The listing builds one solid part. Answer for the finished solid, in the listing's coordinates (mm). Face numbers are marked on the shaded views. A direction names the side the tool comes from. Coordinates: 2 decimals unless noted, no trailing zeros. Write each loop counter-clockwise with the first axis right and the second up, starting at its lowest first coordinate (ties: lowest second). Pieces come first, ordered by that corner, then holes.
(1) Straight lines are drawn through the part: line 1 (X direction, y = -2.05, z = 10.5); line 2 (X direction, y = -4.45, z = 26.5); line 3 (Z direction, x = 48, y = -2.05). For each, find the intervals that lie inside material, in ascending order.
(2) For a pull along X with two mould halves and no side action, classify the marked faces 1, 2, 3 and 4 as +X half, -X half, draft (parallel to the pull), parting line (faces both ways), or undercut.
(3) The part is cut by section C-C on z = 10.25. Determine the outline of the cut face in (x, y), plus the area to 3 significant figures.
(4) Given P1, Ø4, axis at x = 16.5, z = 9.5, coming from the +Y side; P2, Ø10, axis at x = 13.09, z = 10.66, coming from the +Y side, each flat-ended and moving along its own axis, determine where each tip first touches the part or whether it passes through.
(5) The part is cut by section B-B on x = 1.5. Determine the outline of the cut face in (y, z), plus the area to 3 significant figures.
(6) The part is cut by section D-D on x = 32.5. Determine the outline of the cut face in (y, z), plus the area to 3 significant figures.
(7) The part is cut by section A-A on z = 22.25. Determine the outline of the cut face in (x, y).
(8) Which of the six approach directions +Z, -Z, +X, -X, +Y, -Y give full straight-line access (tool end or side, diameter ignored) to the marked faces 5, 6 and 7?
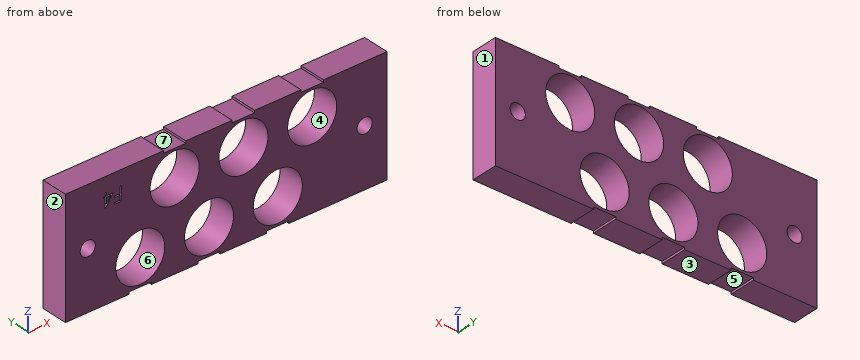
from build123d import *

# Parameters (mm, degrees)
SKETCH1_R               = 5.5
BOSS_EXTRUDE1_DEPTH     = 6
BOSS_EXTRUDE1_2_DEPTH   = 6
BOSS_EXTRUDE1_3_DEPTH   = 6
BOSS_EXTRUDE1_4_DEPTH   = 6
BOSS_EXTRUDE1_5_DEPTH   = 6
BOSS_EXTRUDE1_6_DEPTH   = 6
BOSS_EXTRUDE2_START     = -6
BOSS_EXTRUDE2_OUTLINE_R = 1.7
BOSS_EXTRUDE2_DEPTH     = 6
CUT_EXTRUDE1_DEPTH      = 1


# Read off the part's stored shape, not the designer's step: Boss-Extrude2
with BuildPart() as part:
    # Sketch1 → Boss-Extrude1 (new body)
    with BuildSketch(Plane(origin=(0, 0, 0), x_dir=(1, 0, 0), z_dir=(0, 1, 0))):
        Polygon((3.686387934, -16.664883738), (3.686388262, -4.664883738), (-8.313611738, -4.66488341), (-8.313612066, -16.66488341), align=None)
        with Locations(Location((-2.313611902, -10.664883574, 0), (0, 0, 270))):
            Circle(SKETCH1_R, mode=Mode.SUBTRACT)
    extrude(amount=-BOSS_EXTRUDE1_DEPTH)



with BuildPart() as body_2:
    # Sketch1 → Boss-Extrude1 2 (new body)
    with BuildSketch(Plane(origin=(0, 0, 0), x_dir=(1, 0, 0), z_dir=(0, 1, 0))):
        Polygon((19.086387939, -16.664884095), (19.086388267, -4.664884095), (7.086388267, -4.664883767), (7.086387939, -16.664883767), align=None)
        with Locations(Location((13.086388103, -10.664883931, 0), (0, 0, 270))):
            Circle(SKETCH1_R, mode=Mode.SUBTRACT)
    extrude(amount=-BOSS_EXTRUDE1_2_DEPTH)


with BuildPart() as body_3:
    # Sketch1 → Boss-Extrude1 3 (new body)
    with BuildSketch(Plane(origin=(0, 0, 0), x_dir=(1, 0, 0), z_dir=(0, 1, 0))):
        Polygon((34.486387949, -16.66488445), (34.486388277, -4.66488445), (22.486388277, -4.664884122), (22.486387949, -16.664884122), align=None)
        with Locations(Location((28.486388113, -10.664884286, 0), (0, 0, 270))):
            Circle(SKETCH1_R, mode=Mode.SUBTRACT)
    extrude(amount=-BOSS_EXTRUDE1_3_DEPTH)


with BuildPart() as body_4:
    # Sketch1 → Boss-Extrude1 4 (new body)
    with BuildSketch(Plane(origin=(0, 0, 0), x_dir=(1, 0, 0), z_dir=(0, 1, 0))):
        Polygon((14.786387887, -17.664883977), (14.786387559, -29.664883977), (26.786387559, -29.664884305), (26.786387887, -17.664884305), align=None)
        with Locations(Location((20.786387723, -23.664884141, 0), (0, 0, 270))):
            Circle(SKETCH1_R, mode=Mode.SUBTRACT)
    extrude(amount=-BOSS_EXTRUDE1_4_DEPTH)


with BuildPart() as body_5:
    # Sketch1 → Boss-Extrude1 5 (new body)
    with BuildSketch(Plane(origin=(0, 0, 0), x_dir=(1, 0, 0), z_dir=(0, 1, 0))):
        Polygon((30.186386338, -17.664884333), (30.18638601, -29.664884333), (42.18638601, -29.664884661), (42.186386338, -17.664884661), align=None)
        with Locations(Location((36.186386174, -23.664884497, 0), (0, 0, 270))):
            Circle(SKETCH1_R, mode=Mode.SUBTRACT)
    extrude(amount=-BOSS_EXTRUDE1_5_DEPTH)


with BuildPart() as body_6:
    # Sketch1 → Boss-Extrude1 6 (new body)
    with BuildSketch(Plane(origin=(0, 0, 0), x_dir=(1, 0, 0), z_dir=(0, 1, 0))):
        Polygon((-0.613612103, -17.664883618), (-0.613612431, -29.664883618), (11.386387569, -29.664883947), (11.386387897, -17.664883947), align=None)
        with Locations(Location((5.386387733, -23.664883782, 0), (0, 0, 270))):
            Circle(SKETCH1_R, mode=Mode.SUBTRACT)
    extrude(amount=-BOSS_EXTRUDE1_6_DEPTH)


with BuildPart() as part_1:
    add(part.part)

    add(body_2.part)  # Boss-Extrude2 merges body 2

    add(body_3.part)  # Boss-Extrude2 merges body 3

    add(body_4.part)  # Boss-Extrude2 merges body 4

    add(body_5.part)  # Boss-Extrude2 merges body 5

    add(body_6.part)  # Boss-Extrude2 merges body 6
    # Boss-Extrude2 outline → Boss-Extrude2 (add)
    with BuildSketch(Plane(origin=(0, 0, 0), x_dir=(1, 0, 0), z_dir=(0, 1, 0)).offset(BOSS_EXTRUDE2_START)):
        Polygon((10.586388281, -4.164883862), (0.186388276, -4.164883578), (0.186388262, -4.664883642), (3.686388262, -4.664883738), (3.686387934, -16.664883738), (-8.313612066, -16.66488341), (-8.313611738, -4.66488341), (-4.813611738, -4.664883506), (-4.813611724, -4.164883505), (-19.063611735, -4.164883116), (-19.063612446, -30.164883114), (2.886387555, -30.164883714), (2.886387569, -29.664883714), (-0.613612431, -29.664883618), (-0.613612103, -17.664883618), (11.386387897, -17.664883947), (11.386387569, -29.664883947), (7.886387569, -29.664883851), (7.886387555, -30.164883851), (18.286387545, -30.164884073), (18.286387559, -29.664884073), (14.786387559, -29.664883977), (14.786387887, -17.664883977), (26.786387887, -17.664884305), (26.786387559, -29.664884305), (23.286387559, -29.664884209), (23.286387545, -30.16488421), (33.686385997, -30.164884494), (33.68638601, -29.664884428), (30.18638601, -29.664884333), (30.186386338, -17.664884333), (42.186386338, -17.664884661), (42.18638601, -29.664884661), (38.68638601, -29.664884565), (38.686385997, -30.164884565), (52.936387554, -30.164884954), (52.936388265, -4.164885084), (30.986388291, -4.164884354), (30.986388277, -4.664884354), (34.486388277, -4.66488445), (34.486387949, -16.66488445), (22.486387949, -16.664884122), (22.486388277, -4.664884122), (25.986388277, -4.664884218), (25.986388291, -4.164884218), (15.586388281, -4.164884108), (15.586388267, -4.664883999), (19.086388267, -4.664884095), (19.086387939, -16.664884095), (7.086387939, -16.664883767), (7.086388267, -4.664883767), (10.586388267, -4.664883863), align=None)
        with Locations((47.93638791, -17.164884883)):
            Circle(BOSS_EXTRUDE2_OUTLINE_R, mode=Mode.SUBTRACT)
        with Locations((-14.06361209, -17.164883252)):
            Circle(BOSS_EXTRUDE2_OUTLINE_R, mode=Mode.SUBTRACT)
    extrude(amount=BOSS_EXTRUDE2_DEPTH)

    # Sketch2 → Cut-Extrude1 (cut)
    # profile 1 of 2: a face of its own
    with BuildSketch(Plane(origin=(0, -6, 0), x_dir=(-1, 0, 0), z_dir=(0, -1, 0))):
        Polygon((6.544081332, -23.739762668), (8.090876204, -23.739762668), (8.090876204, -24.065403693), (6.829017229, -24.065403693), (6.829017229, -25.04232677), (8.090876204, -25.04232677), (8.090876204, -25.367967796), (6.829017229, -25.367967796), (6.829017229, -26.914762668), (6.544081332, -26.914762668), align=None)
    # profile 2 of 2: a face of its own
    with BuildSketch(Plane(origin=(0, -6, 0), x_dir=(-1, 0, 0), z_dir=(0, -1, 0))):
        Polygon((10.108960138, -23.658352411), (10.166837742, -23.658352411), (10.166837742, -25.856429335), (10.533183896, -25.856429335), (10.533183896, -26.18207036), (10.166837742, -26.18207036), (10.166837742, -26.914762668), (9.881901845, -26.914762668), (9.881901845, -26.18207036), (8.375812101, -26.18207036), align=None)
        Polygon((9.881901845, -25.856429335), (9.881901845, -24.478815152), (8.936143631, -25.856429335), align=None, mode=Mode.SUBTRACT)
    extrude(amount=-CUT_EXTRUDE1_DEPTH, mode=Mode.SUBTRACT)


solid = part_1.part
Model answer:
1. line 1: x = -19.06 to -7.81, 3.18 to 7.59, 18.58 to 22.99, 33.98 to 52.94
1. line 2: x = -19.06 to 0.67, 10.1 to 16.07, 25.5 to 31.47, 40.9 to 52.94
1. line 3: z = 4.16 to 15.47, 18.86 to 30.16
2. face 1: +X half
2. face 2: -X half
2. face 3: draft
2. face 4: undercut
3. outline: (-19.06, -6) - (-7.8, -6) - (-7.8, 0) - (-19.06, 0) - close; (3.17, -6) - (7.6, -6) - (7.6, 0) - (3.17, 0) - close; (18.57, -6) - (23, -6) - (23, 0) - (18.57, 0) - close; (33.97, -6) - (52.94, -6) - (52.94, 0) - (33.97, 0) - close
3. area: 235 mm2
4. P1: stops at y = 0
4. P2: passes through
5. outline: (-6, 4.16) - (0, 4.16) - (0, 6.7) - (-6, 6.7) - close; (-6, 14.63) - (0, 14.63) - (0, 19.77) - (-6, 19.77) - close; (-6, 27.56) - (0, 27.56) - (0, 30.16) - (-6, 30.16) - close
5. area: 61.7 mm2
6. outline: (-6, 4.16) - (0, 4.16) - (0, 6.9) - (-6, 6.9) - close; (-6, 14.43) - (0, 14.43) - (0, 19.58) - (-6, 19.58) - close; (-6, 27.75) - (0, 27.75) - (0, 30.16) - (-6, 30.16) - close
6. area: 61.9 mm2
7. outline: (-19.06, -6) - (0.07, -6) - (0.07, 0) - (-19.06, 0) - close; (10.7, -6) - (15.47, -6) - (15.47, 0) - (10.7, 0) - close; (26.1, -6) - (30.87, -6) - (30.87, 0) - (26.1, 0) - close; (41.5, -6) - (52.94, -6) - (52.94, 0) - (41.5, 0) - close
8. face 5: -Z, +Y, -Y
8. face 6: +Y, -Y
8. face 7: +Z, +Y, -Y
